CAD build for the part. Positions are in the model's coordinates, mm. Face numbers are marked on the shaded views. A direction names the side the tool comes from. Give positions to 0.01 mm unless a question says otherwise; leave off trailing zeros. Write each loop counter-clockwise with the first axis right and the second up, starting at its lowest first coordinate (ties: lowest second). Pieces come first, ordered by that corner, then holes. Notation, with made-up numbers: (67, -16) - (118, -16) arc R14 ccw to (118, -5) - close; hole circle Ø6 at (16.5, -23). An arc over 180 degrees is marked (long way). Answer as a JSON object with one key per item and string values.
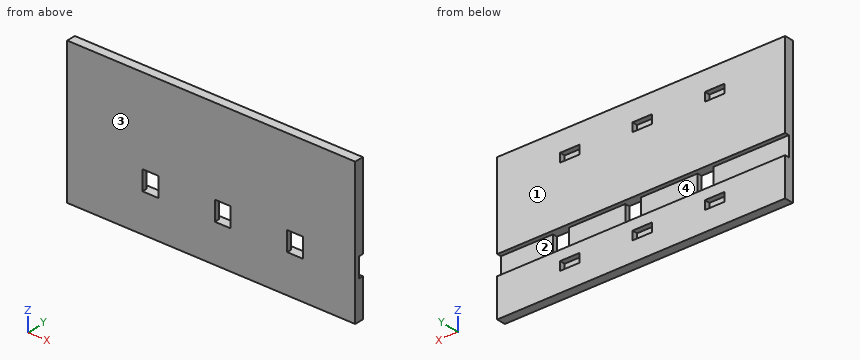
from build123d import *

# Parameters (mm, degrees)
SKETCH1_W                     = 101.092
SKETCH1_H                     = 50.292
BOSS_EXTRUDE1_DEPTH           = 3.175
SKETCH2_W                     = 5.588
SKETCH2_H                     = 6.858
WIRE_HOLE_DEPTH               = 4.175
SKETCH3_W                     = 6.858
SKETCH3_H                     = 3.048
CUT_EXTRUDE2_DEPTH            = 1.905
LPATTERN1_COUNT               = 2
LPATTERN1_PITCH               = 25.4
LPATTERN1_COPY_1_SKETCH_W     = 6.858
LPATTERN1_COPY_1_SKETCH_H     = 3.048
LPATTERN1_COPY_1_DEPTH        = 1.905
LPATTERN1_COL_COUNT           = 2
LPATTERN1_COL_PITCH           = 25.4
LPATTERN1_COL_COPY_1_SKETCH_W = 6.858
LPATTERN1_COL_COPY_1_SKETCH_H = 3.048
LPATTERN1_COL_COPY_1_DEPTH    = 1.905
SKETCH4_W                     = 101.092
SKETCH4_H                     = 6.858
CUT_EXTRUDE3_DEPTH            = 1.524


with BuildPart() as part:
    # Sketch1 → Boss-Extrude1 (new body)
    with BuildSketch(Plane(origin=(0, 0, 0), x_dir=(1, 0, 0), z_dir=(0, 1, 0))):
        Rectangle(SKETCH1_W, SKETCH1_H)
    extrude(amount=BOSS_EXTRUDE1_DEPTH)

    # Sketch2 → Wire Hole (cut, through all)
    with BuildSketch(Plane(origin=(0, 3.175, 0), x_dir=(1, 0, 0), z_dir=(0, 1, 0))):
        with Locations((4.064, 8.322545685)):
            Rectangle(SKETCH2_W, SKETCH2_H)
    wire_hole = extrude(amount=-WIRE_HOLE_DEPTH, mode=Mode.SUBTRACT)

    # Sketch3 → Cut-Extrude2 (cut)
    with BuildSketch(Plane(origin=(0, 3.175, 0), x_dir=(1, 0, 0), z_dir=(0, 1, 0))):
        with Locations((-0.381, 16.764)):
            Rectangle(SKETCH3_W, SKETCH3_H)
    cut_extrude2 = extrude(amount=-CUT_EXTRUDE2_DEPTH, mode=Mode.SUBTRACT)

    # Mirror1: Cut-Extrude2 across plane
    add(cut_extrude2.mirror(Plane.XY), mode=Mode.SUBTRACT)

    # LPattern1: Wire Hole, Cut-Extrude2 ×2
    with Locations(*[(-i * LPATTERN1_PITCH, 0, 0) for i in range(1, LPATTERN1_COUNT)]):
        add(wire_hole, mode=Mode.SUBTRACT)
        add(cut_extrude2, mode=Mode.SUBTRACT)

    # LPattern1 copy 1 sketch → LPattern1 copy 1 (cut)
    with BuildSketch(Plane(origin=(-25.4, 3.175, 0), x_dir=(1, 0, 0), z_dir=(0, 1, 0))):
        with Locations((-0.381, -16.764)):
            Rectangle(LPATTERN1_COPY_1_SKETCH_W, LPATTERN1_COPY_1_SKETCH_H)
    extrude(amount=-LPATTERN1_COPY_1_DEPTH, mode=Mode.SUBTRACT)

    # LPattern1 col: Wire Hole, Cut-Extrude2 ×2
    with Locations(*[(i * LPATTERN1_COL_PITCH, 0, 0) for i in range(1, LPATTERN1_COL_COUNT)]):
        add(wire_hole, mode=Mode.SUBTRACT)
        add(cut_extrude2, mode=Mode.SUBTRACT)

    # LPattern1 col copy 1 sketch → LPattern1 col copy 1 (cut)
    with BuildSketch(Plane(origin=(25.4, 3.175, 0), x_dir=(1, 0, 0), z_dir=(0, 1, 0))):
        with Locations((-0.381, -16.764)):
            Rectangle(LPATTERN1_COL_COPY_1_SKETCH_W, LPATTERN1_COL_COPY_1_SKETCH_H)
    extrude(amount=-LPATTERN1_COL_COPY_1_DEPTH, mode=Mode.SUBTRACT)

    # Sketch4 → Cut-Extrude3 (cut)
    with BuildSketch(Plane(origin=(0, 3.175, 0), x_dir=(1, 0, 0), z_dir=(0, 1, 0))):
        with Locations((0, 8.322545685)):
            Rectangle(SKETCH4_W, SKETCH4_H)
    extrude(amount=-CUT_EXTRUDE3_DEPTH, mode=Mode.SUBTRACT)


solid = part.part
Item 1: Cut at C-C (x = -5.5). Give the cut face in (y, z) (3 decimals), and give its area (3 significant figures).
Entries:
{"outline": "(0, -25.146) - (3.175, -25.146) - (3.175, -11.752) - (1.651, -11.752) - (1.651, -4.894) - (3.175, -4.894) - (3.175, 25.146) - (0, 25.146) - close", "area": "149 mm2"}
Item 2: Flat gauge pins, fed straight in: P1, Ø2, axis at x = 13.5, z = -6.5, coming from the +Y side; P2, Ø1.5, axis at x = -24.5, z = 16.5, coming from the +Y side. Where does each tip first touch, or does it go through?
Entries:
{"P1": "y = 1.65", "P2": "y = 1.27"}
Item 3: Probe line 1 (X direction, y = 2.75, z = 17); line 2 (Z direction, x = 32, y = 2.05); line 3 (Y direction, x = -30.5, z = -8.5). List the from-to ranges inside material, lowest first. Write a range as from..to.
Entries:
{"line 1": "-50.55..-29.21, -22.35..-3.81, 3.05..21.59, 28.45..50.55", "line 2": "-25.15..-11.75, -4.89..25.15", "line 3": "0..1.65"}
Item 4: Cut at A-A (y = 2.5). State how many separate pieces and enclosed holes the cut face has, and give its area (3 significant figures).
Entries:
{"separate pieces": "2", "enclosed holes": "6", "area": "4,270 mm2"}
Item 5: Which spindle directions (+Z, -Z, +X, -X, +Y, -Y) get a long thin tool onto all of the face, cutting with end or side? Do the marked faces 1 and 2. Say none if no direction does.
Entries:
{"face 1": "+Z, -Z, +X, -X, +Y", "face 2": "+X, -X, +Y"}
Item 6: Mould opens along Z. For the marked faces 3 and 4 say: +Z half, -Z half, draft (parallel to the pull), parting line (faces both ways), or undercut.
Entries:
{"face 3": "draft", "face 4": "undercut"}
Item 7: Cut at B-B (x = -26). Give the cut face in (y, z) (3 decimals).
Entries:
{"outline": "(0, -25.146) - (3.175, -25.146) - (3.175, -18.288) - (1.27, -18.288) - (1.27, -15.24) - (3.175, -15.24) - (3.175, -11.752) - (1.651, -11.752) - (1.651, -4.894) - (3.175, -4.894) - (3.175, 15.24) - (1.27, 15.24) - (1.27, 18.288) - (3.175, 18.288) - (3.175, 25.146) - (0, 25.146) - close"}
